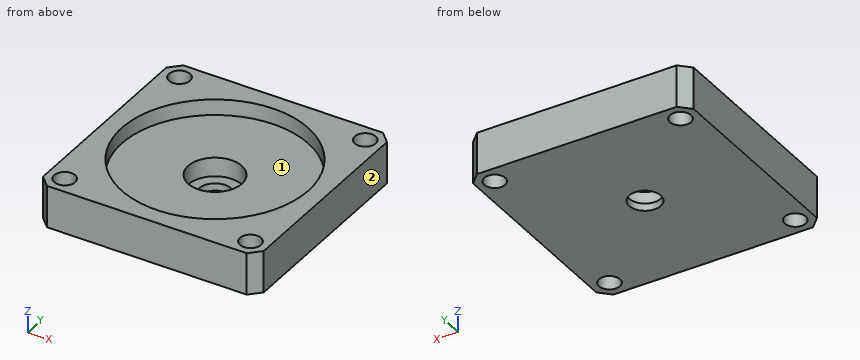
from build123d import *

# Parameters (mm, degrees)
SKETCH_1_W          = 42
SKETCH_1_H          = 42
EXTRUDE_1_DEPTH     = 8
CUT_EXTRUDE_1_REACH = 10
SKETCH_2_R          = 2
SKETCH_3_R          = 17.75
CUT_EXTRUDE_2_DEPTH = 3
SKETCH_4_R          = 5.1
CUT_EXTRUDE_3_DEPTH = 3.6
CUT_EXTRUDE_4_REACH = 3.4
SKETCH_5_R          = 3
CHAMFER_1_SIZE      = 2


with BuildPart() as part:
    # 草图1 → 凸台-拉伸1 (new body)
    with BuildSketch(Plane.XY):
        Rectangle(SKETCH_1_W, SKETCH_1_H)
    extrude(amount=EXTRUDE_1_DEPTH)

    # 草图2 → 切除-拉伸1 (cut, up to next)
    with BuildSketch(Plane.XY.offset(8), mode=Mode.PRIVATE) as cut_extrude_1_sk1:
        with Locations((-17.67766953, 17.67766953)):
            Circle(SKETCH_2_R)
    cut_extrude_1_tool1 = extrude(cut_extrude_1_sk1.sketch, amount=-CUT_EXTRUDE_1_REACH, mode=Mode.PRIVATE) & part.part
    add(cut_extrude_1_tool1.solids().sort_by_distance((-17.67767, 17.67767, 8))[0], mode=Mode.SUBTRACT)
    # 草图2 → 切除-拉伸1 (cut, up to next)
    with BuildSketch(Plane.XY.offset(8), mode=Mode.PRIVATE) as cut_extrude_1_sk2:
        with Locations((17.67766953, 17.67766953)):
            Circle(SKETCH_2_R)
    cut_extrude_1_tool2 = extrude(cut_extrude_1_sk2.sketch, amount=-CUT_EXTRUDE_1_REACH, mode=Mode.PRIVATE) & part.part
    add(cut_extrude_1_tool2.solids().sort_by_distance((17.67767, 17.67767, 8))[0], mode=Mode.SUBTRACT)
    # 草图2 → 切除-拉伸1 (cut, up to next)
    with BuildSketch(Plane.XY.offset(8), mode=Mode.PRIVATE) as cut_extrude_1_sk3:
        with Locations((17.67766953, -17.67766953)):
            Circle(SKETCH_2_R)
    cut_extrude_1_tool3 = extrude(cut_extrude_1_sk3.sketch, amount=-CUT_EXTRUDE_1_REACH, mode=Mode.PRIVATE) & part.part
    add(cut_extrude_1_tool3.solids().sort_by_distance((17.67767, -17.67767, 8))[0], mode=Mode.SUBTRACT)
    # 草图2 → 切除-拉伸1 (cut, up to next)
    with BuildSketch(Plane.XY.offset(8), mode=Mode.PRIVATE) as cut_extrude_1_sk4:
        with Locations((-17.67766953, -17.67766953)):
            Circle(SKETCH_2_R)
    cut_extrude_1_tool4 = extrude(cut_extrude_1_sk4.sketch, amount=-CUT_EXTRUDE_1_REACH, mode=Mode.PRIVATE) & part.part
    add(cut_extrude_1_tool4.solids().sort_by_distance((-17.67767, -17.67767, 8))[0], mode=Mode.SUBTRACT)

    # 草图3 → 切除-拉伸2 (cut)
    with BuildSketch(Plane.XY.offset(8)):
        Circle(SKETCH_3_R)
    extrude(amount=-CUT_EXTRUDE_2_DEPTH, mode=Mode.SUBTRACT)

    # 草图4 → 切除-拉伸3 (cut)
    with BuildSketch(Plane.XY.offset(5)):
        Circle(SKETCH_4_R)
    extrude(amount=-CUT_EXTRUDE_3_DEPTH, mode=Mode.SUBTRACT)

    # 草图5 → 切除-拉伸4 (cut, up to next)
    with BuildSketch(Plane.XY.offset(1.4), mode=Mode.PRIVATE) as cut_extrude_4_sk1:
        Circle(SKETCH_5_R)
    cut_extrude_4_tool1 = extrude(cut_extrude_4_sk1.sketch, amount=-CUT_EXTRUDE_4_REACH, mode=Mode.PRIVATE) & part.part
    add(cut_extrude_4_tool1.solids().sort_by_distance((0, 0, 1.4))[0], mode=Mode.SUBTRACT)

    # 倒角1
    chamfer_1_edges = [part.edges().sort_by_distance(p)[0] for p in [
        (21, -21, 4),
        (-21, -21, 4),
        (-21, 21, 4),
        (21, 21, 4),
    ]]
    chamfer(chamfer_1_edges, length=CHAMFER_1_SIZE)


solid = part.part
Design review of the part built by this model. Coordinates are the model's own, in mm. Face numbers are marked on the shaded views. A direction names the side the tool comes from. Give positions to 0.01 mm unless a question says otherwise; leave off trailing zeros. Loops run counter-clockwise (first coordinate to the right, second up) from the corner with the lowest first, then second, coordinate; pieces in that order, holes last. Notation, with made-up numbers: (74.5, 58) - (90.5, 58) arc R20 cw to (90.5, 85) - close; hole circle Ø3 at (-21, 46.5). An arc over 180 degrees is marked (long way). Write item = value, one per line.
1) Take a section at C-C on z = 2. State the section outline as (x, y) points.
Result sheet:
outline = (-21, -19) - (-19, -21) - (19, -21) - (21, -19) - (21, 19) - (19, 21) - (-19, 21) - (-21, 19) - close; hole circle Ø4 at (-17.68, -17.68); hole circle Ø4 at (-17.68, 17.68); hole circle Ø10.2 at (0, 0); hole circle Ø4 at (17.68, -17.68); hole circle Ø4 at (17.68, 17.68)
2) Take a section at A-A on y = 0. State the section outline as (x, z) points.
Result sheet:
outline = (-21, 0) - (-3, 0) - (-3, 1.4) - (-5.1, 1.4) - (-5.1, 5) - (-17.75, 5) - (-17.75, 8) - (-21, 8) - close; (3, 0) - (21, 0) - (21, 8) - (17.75, 8) - (17.75, 5) - (5.1, 5) - (5.1, 1.4) - (3, 1.4) - close
3) Clearance check with flat-ended pins moving along their axes: pin 1 Ø2.5 at (x, y) = (17.68, -17.68) entering from -Z; pin 2 Ø10 at (x, y) = (-7.5, -0.5) entering from +Z; pin 3 Ø3 at (x, y) = (2, 1) entering from +Z. State where each tip first meets the part, or that it passes through.
Result sheet:
pin_1 = through
pin_2 = 5
pin_3 = 1.4
4) Tool access review of the marked faces 1 and 2: name each direction out of +Z, -Z, +X, -X, +Y, -Y from which nothing blocks a thin tool from reaching the whole face with its end or side.
Result sheet:
face_1 = +Z
face_2 = +Z, -Z, +X, +Y, -Y
5) Take a section at D-D on x = 17. State the section outline as (y, z) points.
Result sheet:
outline = (-21, 0) - (-19.56, 0) - (-19.56, 8) - (-21, 8) - close; (-15.8, 0) - (15.8, 0) - (15.8, 8) - (5.11, 8) - (5.11, 5) - (-5.11, 5) - (-5.11, 8) - (-15.8, 8) - close; (19.56, 0) - (21, 0) - (21, 8) - (19.56, 8) - close
6) To check wall thickness, follow line 1 (Y direction, x = 17.5, z = 0.5); line 2 (Y direction, x = 0, z = 2); line 3 (Y direction, x = 17, z = 3.25). State the ranges of each line that lie inside material, in increasing order.
Result sheet:
line_1 = -21 to -19.67, -15.69 to 15.69, 19.67 to 21
line_2 = -21 to -5.1, 5.1 to 21
line_3 = -21 to -19.56, -15.8 to 15.8, 19.56 to 21
